Part print with two shaded views. Sizes in mm from the minimum x, y, z corner. A direction names the side the tool comes from. Round coordinates to 2 decimals unless told otherwise and drop trailing zeros. Write each loop counter-clockwise with the first axis right and the second up, starting at its lowest first coordinate (ties: lowest second). Pieces come first, ordered by that corner, then holes. Notation, with made-up numbers: (30, 86) - (89, 86) arc R26 ccw to (89, 123) - close; hole circle Ø5 at (-2, 23). An arc over 180 degrees is marked (long way). Answer as a JSON object with one key per item and string values. Group by question number.
Item 1: Slice it at B-B, the plane y = 5. List the corners of the cut face in (x, z), then the cut area to 3 significant figures.
Item 2: Slice it at A-A, the plane x = 66.5. List the corners of the cut face in (y, z).
Item 3: Probe line 1 (Y direction, x = 66, z = 9.5); line 2 (X direction, y = 18.5, z = 4); line 3 (X direction, y = 3, z = 8.5). List the from-to ranges inside material, lowest first. Write a range as from..to.
Item 4: Which spindle directions (+Z, -Z, +X, -X, +Y, -Y) get a long thin tool onto all of the face, cutting with end or side? Do the marked faces 4 and 5. Say none if no direction does.
Item 5: Slice it at C-C, the plane z = 3. List the corners of the cut face in (x, y).
Item 6: Slice it at D-D, the plane y = 12. List the corners of the cut face in (x, z), then the cut area to 3 significant figures.
Item 7: Flat gauge pins, fed straight in: pin 1 (0.9 mm diameter, centred on x = 84, z = 3.5, fed in from -Y); pin 2 (3.5 mm diameter, centred on x = 84.5, z = 3.5, fed in from +Y). Where does each tip first touch, or does it go through?
Item 8: Two-plate mould, pull along X, no slides. Class the marked faces 1, 2 and 3: +X half, -X half, draft (parallel to the pull), parting line (faces both ways), or undercut.
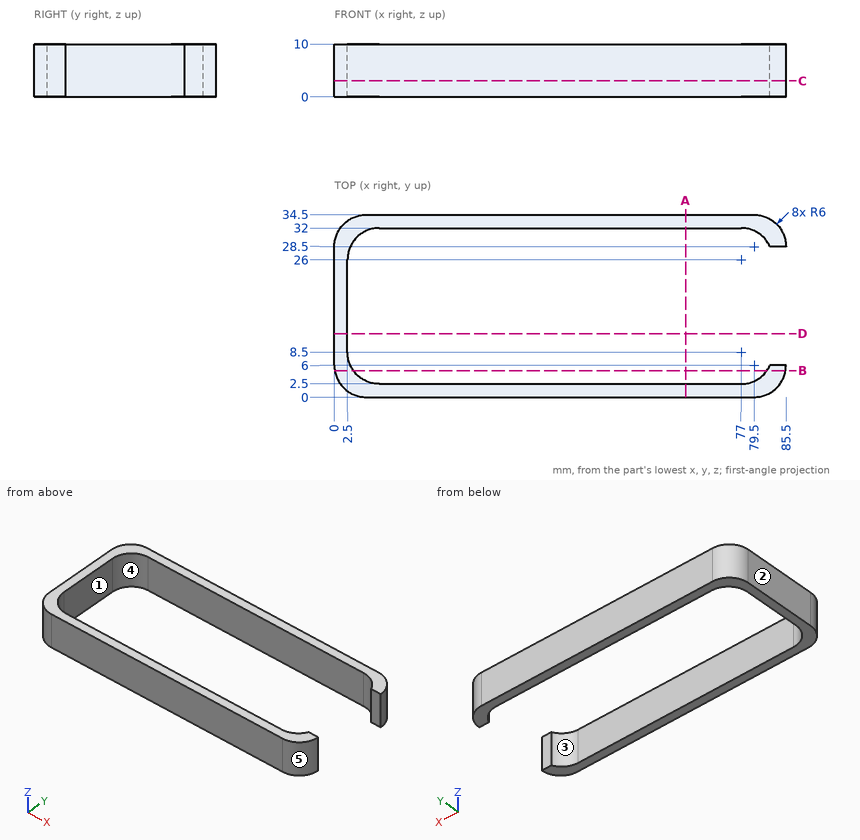
Geometry says:
{
 "1": {"outline": "(0.08, 0) - (3.63, 0) - (3.63, 10) - (0.08, 10) - close; (81.87, 0) - (85.42, 0) - (85.42, 10) - (81.87, 10) - close", "area": "70.9 mm^2"},
 "2": {"outline": "(0, 0) - (2.5, 0) - (2.5, 10) - (0, 10) - close; (32, 0) - (34.5, 0) - (34.5, 10) - (32, 10) - close"},
 "3": {"line 1": "y = 0..2.5, 32..34.5", "line 2": "x = 0..2.5", "line 3": "x = 0.8..6.1, 79.4..84.7"},
 "4": {"face 4": "+Z, -Z", "face 5": "+Z, -Z, +X, -Y"},
 "5": {"outline": "(0, 6) arc R6 ccw to (6, 0) - (79.5, 0) arc R6 ccw to (85.5, 6) - (82.45, 6) arc R6 cw to (77, 2.5) - (8.5, 2.5) arc R6 cw to (2.5, 8.5) - (2.5, 26) arc R6 cw to (8.5, 32) - (77, 32) arc R6 cw to (82.45, 28.5) - (85.5, 28.5) arc R6 ccw to (79.5, 34.5) - (6, 34.5) arc R6 ccw to (0, 28.5) - close"},
 "6": {"outline": "(0, 0) - (2.5, 0) - (2.5, 10) - (0, 10) - close", "area": "25.0 mm^2"},
 "7": {"pin 1": "stops at y = 1.57", "pin 2": "stops at y = 33.54"},
 "8": {"face 1": "+X half", "face 2": "-X half", "face 3": "undercut"}
}
